For this review, take the finished solid that the model builds, in its own axes (mm). A direction names the side the tool comes from. Give positions to 0.01 mm unless a question says otherwise; leave off trailing zeros. Order: outer loops, then holes, each group sorted by start corner. A loop starts at its lowest first (then second) coordinate and runs counter-clockwise, first axis right, second up.
from build123d import *

# Parameters (mm, degrees)
F0_W     = 40
F0_H     = 40
F0_R     = 18
F1_DEPTH = 10
F2_DEPTH = 9
F3_D     = 4.2
F4_R     = 4


with BuildPart() as f1:
    # F0 (on Top) → F1 (new body)
    with BuildSketch(Plane.XY):
        Rectangle(F0_W, F0_H)
        Circle(F0_R, mode=Mode.SUBTRACT)
    extrude(amount=F1_DEPTH)

    # F0 (on Top) → F2 (join)
    with BuildSketch(Plane.XY):
        Circle(F0_R)
    extrude(amount=F2_DEPTH)

    # F3 (through all)
    with Locations(Plane(origin=(0, 0, 0), x_dir=(1, 0, 0), z_dir=(0, 0, -1))):
        with Locations((-16, 16), (-16, -16), (16, -16), (16, 16)):
            Hole(F3_D / 2)

    # F4
    f4_edges = [f1.edges().sort_by_distance(p)[0] for p in [
        (-20, -20, 5),
        (-20, 20, 5),
        (20, 20, 5),
        (20, -20, 5),
    ]]
    fillet(f4_edges, radius=F4_R)


solid = f1.part
1) We need section C-C on y = 14.5. Give the boundary of the cut face in (x, z).
Answer sheet:
outline: (-20, 0) - (-17.47, 0) - (-17.47, 10) - (-20, 10) - close; (-14.53, 0) - (14.53, 0) - (14.53, 10) - (10.67, 10) - (10.67, 9) - (-10.67, 9) - (-10.67, 10) - (-14.53, 10) - close; (17.47, 0) - (20, 0) - (20, 10) - (17.47, 10) - close
2) We need section B-B on x = -15.5. Give the boundary of the cut face in (y, z), then the cut area to 3 significant figures.
Answer sheet:
outline: (-20, 0) - (-18.04, 0) - (-18.04, 10) - (-20, 10) - close; (-13.96, 0) - (13.96, 0) - (13.96, 10) - (9.15, 10) - (9.15, 9) - (-9.15, 9) - (-9.15, 10) - (-13.96, 10) - close; (18.04, 0) - (20, 0) - (20, 10) - (18.04, 10) - close
area: 300 mm2
3) To check wall thickness, follow line 1 (X direction, y = -16, z = 5); line 2 (Y direction, x = 0, z = 9.75). State the ranges of each line that lie inside material, in increasing order.
Answer sheet:
line 1: x = -20 to -18.1, -13.9 to 13.9, 18.1 to 20
line 2: y = -20 to -18, 18 to 20
4) Tool access review of faces 1 (the face through (-2.343, 17.847, 9.493)), 2 (the face through (0, 20, 5)): name each direction out of +Z, -Z, +X, -X, +Y, -Y from which nothing blocks a thin tool from reaching the whole face with its end or side.
Answer sheet:
face 1: +Z
face 2: +Z, -Z, +X, -X, +Y
5) We need section A-A on z = 1. Give the boundary of the cut face in (x, y).
Answer sheet:
outline: (-20, -16) arc R4 ccw to (-16, -20) - (16, -20) arc R4 ccw to (20, -16) - (20, 16) arc R4 ccw to (16, 20) - (-16, 20) arc R4 ccw to (-20, 16) - close; hole circle Ø4.2 at (-16, -16); hole circle Ø4.2 at (-16, 16); hole circle Ø4.2 at (16, -16); hole circle Ø4.2 at (16, 16)
6) Draft analysis for pull direction X (two halves, no side actions). For faces 3 (the face through (-20, 0, 5)), 4 (the face through (-15.727, 13.918, 5.07)), 5 (the face through (20, 0, 5)), 6 (the face through (0, -20, 5)), state which applies: +X half, -X half, draft (parallel to the pull), parting line (faces both ways), or undercut.
Answer sheet:
face 3: -X half
face 4: undercut
face 5: +X half
face 6: draft
7) We need section D-D on y = 0. Give the boundary of the cut face in (x, z), then the cut area to 3 significant figures.
Answer sheet:
outline: (-20, 0) - (20, 0) - (20, 10) - (18, 10) - (18, 9) - (-18, 9) - (-18, 10) - (-20, 10) - close
area: 364 mm2
